Verification items for the finished model (mm, model axes). Round coordinates to 2 decimals unless told otherwise and drop trailing zeros. Loops run counter-clockwise (first coordinate to the right, second up) from the corner with the lowest first, then second, coordinate; pieces in that order, holes last. Notation, with made-up numbers: (22.5, 9) -> (60.5, 9) arc R17 ccw to (60.5, 26) -> close; hole circle Ø3 at (83, -29.5). An arc over 180 degrees is marked (long way). Write item = value, one per line.
```python
from build123d import *

# Parameters (mm, degrees)
BOSS_EXTRUDE1_DEPTH      = 19.05
BOSS_EXTRUDE1_DEPTH_BACK = 4.191
SKETCH2_W                = 87.253712628
SKETCH2_H                = 39.813319923
CUT_EXTRUDE1_DEPTH       = 4.24112422
CUT_EXTRUDE1_DEPTH_BACK  = 8.248720327
SKETCH3_W                = 1.428322818
SKETCH3_H                = 1.598014705
CUT_EXTRUDE2_DEPTH       = 19.05
CUT_EXTRUDE2_DEPTH_BACK  = 19.05
CUT_EXTRUDE3_DEPTH       = 1.219470239
CUT_EXTRUDE3_DEPTH_BACK  = 8.664708383


with BuildPart() as part:
    # Sketch1 → Boss-Extrude1 (new body, two sides)
    with BuildSketch(Plane.XY) as boss_extrude1_sk:
        with BuildLine():
            Line((-75.189237024, -5.096374737), (-73.665237024, -5.043705171))
            ThreePointArc((-73.665237024, -5.043705171), (-42.636952293, 0.217377617), (-11.542527873, -4.637539006))
            Line((-11.542527873, -4.637539006), (-12.016580594, -6.085934677))
            ThreePointArc((-12.016580594, -6.085934677), (-42.739704949, -1.307392681), (-73.385520331, -6.558947999))
            Line((-73.385520331, -6.558947999), (-74.965667148, -6.613558005))
            ThreePointArc((-74.965667148, -6.613558005), (-81.004050329, -7.593414774), (-87.118989346, -7.421044375))
            Line((-87.118989346, -7.421044375), (-86.932454331, -5.908503239))
            ThreePointArc((-86.932454331, -5.908503239), (-81.021793865, -6.067120464), (-75.189237024, -5.096374737))
        make_face()
    extrude(amount=BOSS_EXTRUDE1_DEPTH)
    extrude(boss_extrude1_sk.sketch, amount=-BOSS_EXTRUDE1_DEPTH_BACK)

    # Sketch2 → Cut-Extrude1 (cut, two sides)
    with BuildSketch(Plane(origin=(0.138860316, -4.017939298, 0), x_dir=(-0.999403335, -0.034539462, 0), z_dir=(0.034539462, -0.999403335, 0))) as cut_extrude1_sk:
        with Locations((49.508356896, -7.260136502)):
            Rectangle(SKETCH2_W, SKETCH2_H)
        with BuildLine():
            Line((42.893945954, -19.05), (58.535995628, -19.05))
            ThreePointArc((58.535995628, -19.05), (75.136021198, -14.244685293), (87.323327356, -1.992278715))
            ThreePointArc((87.323327356, -1.992278715), (85.416060887, 2.217888864), (81.236346917, 4.191))
            Line((81.236346917, 4.191), (42.893945954, 4.191))
            ThreePointArc((42.893945954, 4.191), (26.378637692, 0.840637304), (11.695818951, -7.4295))
            ThreePointArc((11.695818951, -7.4295), (26.325842273, -15.841379758), (42.893945954, -19.05))
        make_face(mode=Mode.SUBTRACT)
    extrude(amount=CUT_EXTRUDE1_DEPTH, mode=Mode.SUBTRACT)
    extrude(cut_extrude1_sk.sketch, amount=-CUT_EXTRUDE1_DEPTH_BACK, mode=Mode.SUBTRACT)

    # Sketch3 → Cut-Extrude2 (cut, two sides)
    with BuildSketch(Plane(origin=(0.138860316, -4.017939298, 0), x_dir=(0.999403335, 0.034539462, 0), z_dir=(0.034539462, -0.999403335, 0))) as cut_extrude2_sk:
        with Locations((-74.593800237, -0.799007353)):
            Rectangle(SKETCH3_W, SKETCH3_H)
    extrude(amount=CUT_EXTRUDE2_DEPTH, mode=Mode.SUBTRACT)
    extrude(cut_extrude2_sk.sketch, amount=-CUT_EXTRUDE2_DEPTH_BACK, mode=Mode.SUBTRACT)

    # Sketch4 → Cut-Extrude3 (cut, two sides)
    with BuildSketch(Plane(origin=(0, 0, 0), x_dir=(1, 0, 0), z_dir=(0, 1, 0))) as cut_extrude3_sk:
        with BuildLine():
            Line((-64.893542216, -6.597323199), (-53.662481079, -7.351648201))
            ThreePointArc((-53.662481079, -7.351648201), (-52.851129929, -6.642425168), (-53.560352962, -5.831074017))
            Line((-53.560352962, -5.831074017), (-64.791414099, -5.076749016))
            ThreePointArc((-64.791414099, -5.076749016), (-65.60276525, -5.785972049), (-64.893542216, -6.597323199))
        make_face()
        with BuildLine():
            Line((-48.16351423, -7.353361109), (-34.166594754, -7.353361109))
            ThreePointArc((-34.166594754, -7.353361109), (-33.404594754, -6.591361109), (-34.166594754, -5.829361109))
            Line((-34.166594754, -5.829361109), (-48.16351423, -5.829361109))
            ThreePointArc((-48.16351423, -5.829361109), (-48.92551423, -6.591361109), (-48.16351423, -7.353361109))
        make_face()
        with BuildLine():
            ThreePointArc((-68.534997951, -12.362450574), (-60.444707089, -13.294377363), (-52.352141863, -12.382411445))
            ThreePointArc((-52.352141863, -12.382411445), (-38.341637279, -11.721973531), (-24.464171754, -9.685710393))
            ThreePointArc((-24.464171754, -9.685710393), (-23.864251009, -8.790510359), (-24.759451042, -8.190589614))
            ThreePointArc((-24.759451042, -8.190589614), (-38.575832063, -10.213483586), (-52.524637961, -10.857920208))
            ThreePointArc((-52.524637961, -10.857920208), (-60.356328328, -11.770376603), (-68.190325048, -10.877938334))
            ThreePointArc((-68.190325048, -10.877938334), (-69.104917619, -11.447858003), (-68.534997951, -12.362450574))
        make_face()
        with BuildLine():
            ThreePointArc((-25.724196054, -3.936751805), (-38.706541391, -1.164656942), (-51.978446223, -0.877703144))
            ThreePointArc((-51.978446223, -0.877703144), (-60.183282807, 0.29192564), (-68.463888537, -0.052956388))
            ThreePointArc((-68.463888537, -0.052956388), (-69.117907874, -0.9094298), (-68.261434462, -1.563449137))
            ThreePointArc((-68.261434462, -1.563449137), (-60.142415983, -1.236181897), (-52.102798554, -2.415213913))
            ThreePointArc((-52.102798554, -2.415213913), (-39.000033907, -2.664871884), (-26.181471193, -5.390531516))
            ThreePointArc((-26.181471193, -5.390531516), (-25.225943768, -4.892279229), (-25.724196054, -3.936751805))
        make_face()
    extrude(amount=CUT_EXTRUDE3_DEPTH, mode=Mode.SUBTRACT)
    extrude(cut_extrude3_sk.sketch, amount=-CUT_EXTRUDE3_DEPTH_BACK, mode=Mode.SUBTRACT)


solid = part.part
```
(1) Sectioned sample at A-A, the plane x = -46. Record the cut outline in (y, z), and give its area (3 significant figures).
Filled sheet:
outline = (-1.39, -4.19) -> (0.14, -4.19) -> (0.14, 0.7) -> (-1.39, 0.7) -> close; (-1.39, 2.22) -> (0.14, 2.22) -> (0.14, 5.83) -> (-1.39, 5.83) -> close; (-1.39, 7.35) -> (0.14, 7.35) -> (0.14, 10.73) -> (-1.39, 10.73) -> close; (-1.39, 12.25) -> (0.14, 12.25) -> (0.14, 19.05) -> (-1.39, 19.05) -> close
area = 28.5 mm2
(2) Sectioned sample at B-B, the plane z = -2.5. Record the cut outline in (x, y), and give its area (3 significant figures).
Filled sheet:
outline = (-84.96, -6.09) -> (-84.91, -7.62) arc R32.41 ccw to (-74.97, -6.61) -> (-73.39, -6.56) arc R96.38 cw to (-31.59, -1.87) -> (-31.65, -0.33) arc R97.91 ccw to (-73.67, -5.04) -> (-75.19, -5.1) arc R30.88 cw to start
area = 82.3 mm2
(3) Sectioned sample at C-C, the plane x = -31.5. Count the separate pieces of the cut face and the enclosed holes in it, and give its area (3 significant figures).
Filled sheet:
separate_pieces = 3
enclosed_holes = 0
area = 25.8 mm2
(4) Draft check along Z on faces 1 (the face through (-26.195, -2.09, 15.814)), 2 (the face through (-38.522, -0.917, 1.186)), 3 (the face through (-87.006, -6.507, 1.532)). Enter one of: released by +Z, released by -Z, zero draft, split by the parting line, or undercut.
Filled sheet:
face_1 = released by +Z
face_2 = undercut
face_3 = zero draft
(5) Go/stop test with flat-tipped pins: pin 1 Ø6 at (x, z) = (-76, -1) entering from -Y; pin 2 Ø1.6 at (x, y) = (-74.5, -6) entering from +Z; pin 3 Ø1 at (x, z) = (-77.5, 10.5) entering from +Y. Record where each tip stops, or that it passes through.
Filled sheet:
pin_1 = -7.4
pin_2 = 14.96
pin_3 = -5.52
(6) Material ranges on probe 1 along Z at (x, y) = (-37, -0.25); probe 2 along Z at (x, y) = (-62, -2.5); probe 3 along Y at (x, z) = (-76.5, 2.5), recorded low to high. Write a range as from..to.
Filled sheet:
probe_1 = -3.61..1.38, 2.92..5.83, 7.35..10.05, 11.59..18.55
probe_2 = -4.19..-0.35, 1.18..5.26, 6.79..11.73, 13.26..18.77
probe_3 = -6.97..-5.42
